from build123d import *

# Parameters (mm, degrees)
SKETCH1_R               = 3.96875
SKETCH1_R_2             = 3.175
BOSS_EXTRUDE1_DEPTH     = 12.7
CUT_EXTRUDE1_DEPTH      = 120.685287839
CUT_EXTRUDE1_DEPTH_BACK = 120.685287839
SKETCH2_W               = 25.4
SKETCH2_H               = 12.7
SKETCH2_W_2             = 19.05
FILLET1_R               = 1.5875
FILLET2_R               = 1.5875
CUT_EXTRUDE2_DEPTH      = 12.7
CUT_EXTRUDE3_START      = -12.7
CUT_EXTRUDE3_DEPTH      = 12.7


with BuildPart() as part:
    # Sketch1 → Boss-Extrude1 (new, symmetric)
    with BuildSketch(Plane(origin=(0, 0, 0), x_dir=(1, 0, 0), z_dir=(0, 1, 0))):
        with BuildLine():
            Line((-117.475, 12.7), (-101.6, 12.7))
            Line((-101.6, 12.7), (0.370986014, 7.928825615))
            ThreePointArc((0.370986014, 7.928825615), (7.933719481, 0.24495193), (0.859414796, -7.890837247))
            Line((0.859414796, -7.890837247), (-101.6, -19.05))
            Line((-101.6, -19.05), (-117.475, -19.05))
            Line((-117.475, -19.05), (-117.475, 12.7))
        make_face()
        with Locations(Location((0, 0, 0), (0, 0, 270))):
            Circle(SKETCH1_R, mode=Mode.SUBTRACT)
        with Locations(Location((-107.95, 6.35, 0), (0, 0, 270))):
            Circle(SKETCH1_R_2, mode=Mode.SUBTRACT)
        with Locations(Location((-107.95, -12.7, 0), (0, 0, 270))):
            Circle(SKETCH1_R_2, mode=Mode.SUBTRACT)
    extrude(amount=BOSS_EXTRUDE1_DEPTH, both=True)

    # Sketch2 → Cut-Extrude1 (cut, two sides: drawn at the far end of the back side and taken through both)
    with BuildSketch(Plane.XY.offset(-CUT_EXTRUDE1_DEPTH_BACK)):
        Rectangle(SKETCH2_W, SKETCH2_H)
        with Locations((-111.125, 0)):
            Rectangle(SKETCH2_W_2, SKETCH2_H)
    extrude(amount=CUT_EXTRUDE1_DEPTH + CUT_EXTRUDE1_DEPTH_BACK, mode=Mode.SUBTRACT)

    # Fillet1
    fillet1_edges = [part.edges().sort_by_distance(p)[0] for p in [
        (-12.7, -6.35, 0.413611484),
        (-12.7, 6.35, 0.413611484),
        (-101.6, -6.35, 3.175),
        (-101.6, 6.35, 3.175),
    ]]
    fillet(fillet1_edges, radius=FILLET1_R)

    # Fillet2
    fillet2_edges = [part.edges().sort_by_distance(p)[0] for p in [
        (-117.475, 6.35, 3.175),
        (-117.475, -6.35, 3.175),
    ]]
    fillet(fillet2_edges, radius=FILLET2_R)

    # Sketch3 → Cut-Extrude2 (cut)
    with BuildSketch(Plane(origin=(0, 0, -12.7), x_dir=(-1, 0, 0), z_dir=(0, 0, -1))):
        with BuildLine():
            Line((28.575, 6.35), (85.725, 6.35))
            ThreePointArc((85.725, 6.35), (92.075, 0), (85.725, -6.35))
            Line((85.725, -6.35), (28.575, -6.35))
            ThreePointArc((28.575, -6.35), (22.225, 0), (28.575, 6.35))
        make_face()
    extrude(amount=-CUT_EXTRUDE2_DEPTH, mode=Mode.SUBTRACT)

    # Sketch4 → Cut-Extrude3 (cut)
    with BuildSketch(Plane.XY.offset(19.05).offset(CUT_EXTRUDE3_START)):
        with BuildLine():
            Line((-28.575, 6.35), (-85.725, 6.35))
            ThreePointArc((-85.725, 6.35), (-92.075, 0), (-85.725, -6.35))
            Line((-85.725, -6.35), (-28.575, -6.35))
            ThreePointArc((-28.575, -6.35), (-22.225, 0), (-28.575, 6.35))
        make_face()
    extrude(amount=CUT_EXTRUDE3_DEPTH, mode=Mode.SUBTRACT)


solid = part.part
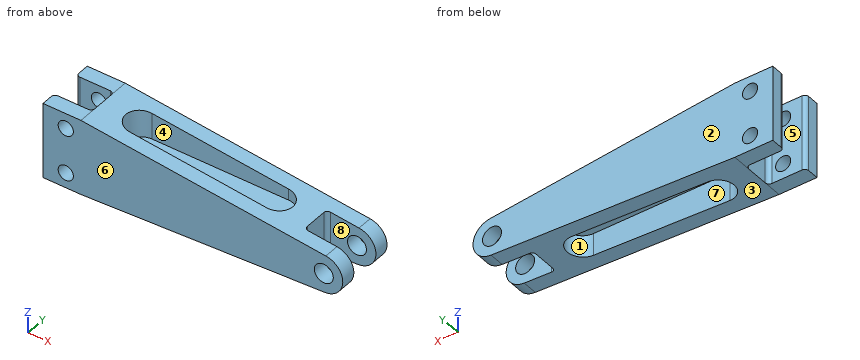
Check sheet for the modelled part. Datum: model origin and axes. Units: mm. Face numbers are marked on the shaded views. A direction names the side the tool comes from. Coordinates: 2 decimals unless noted, no trailing zeros. Loops run counter-clockwise (first coordinate to the right, second up) from the corner with the lowest first, then second, coordinate; pieces in that order, holes last. Notation, with made-up numbers: (32, -17.75) -> (38, -17.75) arc R21 ccw to (38, 9.25) -> close; hole circle Ø10 at (7.25, 6.25). An arc over 180 degrees is marked (long way). Write item = value, one per line. Start each with the question number.
1. Section check A-A on z = -6.35. Give the number of separate pieces and of enclosed holes in the cut face, then the cut area to 3 significant figures.
2. Section check B-B on x = -107.95. Record the cut outline in (y, z) (3 decimals), then the cut area to 3 significant figures.
3. Tool access check on the marked faces 4, 5, 6, 7 and 8. Record the directions out of +Z, -Z, +X, -X, +Y, -Y that give a thin tool (end or side, any length) a straight path to the whole face; none if there is none.
4. Depth check by flat-ended pin: P1, Ø1, axis at x = -89, y = 10, coming from the +Z side; P2, Ø5, axis at y = 7, z = -4, coming from the +X side; P3, Ø3, axis at y = -1.5, z = 6, coming from the -X side. Enter the tip coordinate at first touch or a pass-through.
5. Material ranges on line 1 (Z direction, x = -107.95, y = -9.75) (3 decimals); line 2 (Y direction, x = -83.5, z = 13); line 3 (X direction, y = 8.5, z = 0) (1 decimal), recorded low to high.
6. Draft check along X on the marked faces 1, 2 and 3. Enter one of: released by +X, released by -X, zero draft, split by the parting line, or undercut.
Responses:
q1.separate_pieces = 3
q1.enclosed_holes = 1
q1.area = 1,750 mm2
q2.outline = (-12.7, -12.7) -> (-6.35, -12.7) -> (-6.35, -9.525) -> (-12.7, -9.525) -> close; (-12.7, -3.175) -> (-6.35, -3.175) -> (-6.35, 9.525) -> (-12.7, 9.525) -> close; (-12.7, 15.875) -> (-6.35, 15.875) -> (-6.35, 19.05) -> (-12.7, 19.05) -> close; (6.35, -12.7) -> (12.7, -12.7) -> (12.7, -9.525) -> (6.35, -9.525) -> close; (6.35, -3.175) -> (12.7, -3.175) -> (12.7, 9.525) -> (6.35, 9.525) -> close; (6.35, 15.875) -> (12.7, 15.875) -> (12.7, 19.05) -> (6.35, 19.05) -> close
q2.area = 242 mm2
q3.face_4 = +Z
q3.face_5 = +Z, -Z, -X
q3.face_6 = +Z, -Z, +X, -X, -Y
q3.face_7 = -Z
q3.face_8 = +Z, -Z, +X
q4.P1 = 17.73
q4.P2 = 7.79
q4.P3 = -101.6
q5.line_1 = -12.7 to -9.525, -3.175 to 9.525, 15.875 to 19.05
q5.line_2 = -12.7 to -6.35, 6.35 to 12.7
q5.line_3 = -117.5 to -4, 4 to 7.9
q6.face_1 = undercut
q6.face_2 = zero draft
q6.face_3 = released by +X
